```python
from build123d import *

# Parameters (mm, degrees)
SKETCH1_R           = 1.5
BOSS_EXTRUDE1_DEPTH = 3
SKETCH3_W           = 11
SKETCH3_H           = 6
CUT_EXTRUDE2_DEPTH  = 1


with BuildPart() as part:
    # Sketch1 → Boss-Extrude1 (new body)
    with BuildSketch(Plane(origin=(0, 0, 0), x_dir=(0, 0, -1), z_dir=(1, 0, 0))):
        with BuildLine():
            Line((0, 3), (40.5, 3))
            ThreePointArc((40.5, 3), (43.5, 0), (40.5, -3))
            Line((40.5, -3), (0, -3))
            ThreePointArc((0, -3), (-3, 0), (0, 3))
        make_face()
        Circle(SKETCH1_R, mode=Mode.SUBTRACT)
        with Locations((40.5, 0)):
            Circle(SKETCH1_R, mode=Mode.SUBTRACT)
    extrude(amount=BOSS_EXTRUDE1_DEPTH)

    # Sketch3 → Cut-Extrude2 (cut)
    with BuildSketch(Plane.ZY):
        with Locations((-38, 0)):
            Rectangle(SKETCH3_W, SKETCH3_H)
    extrude(amount=-CUT_EXTRUDE2_DEPTH, mode=Mode.SUBTRACT)


solid = part.part
```
Read the model definition and answer for the solid it produces. Units are mm, in the model's axes. A direction names the side the tool comes from. Coordinates: 2 decimals unless noted, no trailing zeros. Write each loop counter-clockwise with the first axis right and the second up, starting at its lowest first coordinate (ties: lowest second). Pieces come first, ordered by that corner, then holes. Notation, with made-up numbers: (3, 32.5) -> (12, 32.5) arc R9 ccw to (12, 39.5) -> close; hole circle Ø2 at (-1, -9). An arc over 180 degrees is marked (long way). Write item = value, one per line.
(1) Section B-B on x = 2.05 is taken. Write down the section's boundary in (y, z).
From the geometry:
outline = (-3, -40.5) arc R3 ccw to (3, -40.5) -> (3, 0) arc R3 ccw to (-3, 0) -> close; hole circle Ø3 at (0, -40.5); hole circle Ø3 at (0, 0)
(2) Given pin 1 Ø0.8 at (x, y) = (0.5, 1) entering from -Z; pin 2 Ø1.5 at (x, y) = (1.5, -1.5) entering from -Z, each flat-ended and moving along its own axis, determine where each tip first touches the part or whether it passes through.
From the geometry:
pin_1 = -32.5
pin_2 = -43.4
(3) Section A-A on y = 0 is taken. Write down the section's boundary in (x, z), plus the area to 4 significant figures.
From the geometry:
outline = (0, -32.5) -> (1, -32.5) -> (1, -39) -> (3, -39) -> (3, -1.5) -> (0, -1.5) -> close; (0, 1.5) -> (3, 1.5) -> (3, 3) -> (0, 3) -> close; (1, -43.5) -> (3, -43.5) -> (3, -42) -> (1, -42) -> close
area = 113.5 mm2
(4) Straight lines are drawn through the part: L1, parallel to Y at x = 1, z = 0; L2, parallel to Z at x = 1.6, y = 1.3; L3, parallel to Z at x = 2.85, y = 1.1. For each, find the intervals that lie inside material, in ascending order. Write a range as from..to.
From the geometry:
L1 = -3..-1.5, 1.5..3
L2 = -43.2..-41.25, -39.75..-0.75, 0.75..2.7
L3 = -43.29..-41.52, -39.48..-1.02, 1.02..2.79
(5) For a pull along Y with two mould halves and no side action, classify faces 1 (the face through (2, 0, -39)), 2 (the face through (0.5, 0, -32.5)), 3 (the face through (1, 3, -20)) as +Y half, -Y half, draft (parallel to the pull), parting line (faces both ways), or undercut.
From the geometry:
face_1 = undercut
face_2 = draft
face_3 = +Y half
(6) Section C-C on z = -34 is taken. Write down the section's boundary in (x, y).
From the geometry:
outline = (1, -3) -> (3, -3) -> (3, 3) -> (1, 3) -> close
(7) Which of the six approach directions +Z, -Z, +X, -X, +Y, -Y give full straight-line access (tool end or side, diameter ignored) to faces 4 (the face through (0, 0, -15)), 5 (the face through (1, 0, -37))?
From the geometry:
face_4 = +Z, -Z, -X, +Y, -Y
face_5 = -Z, -X, +Y, -Y
